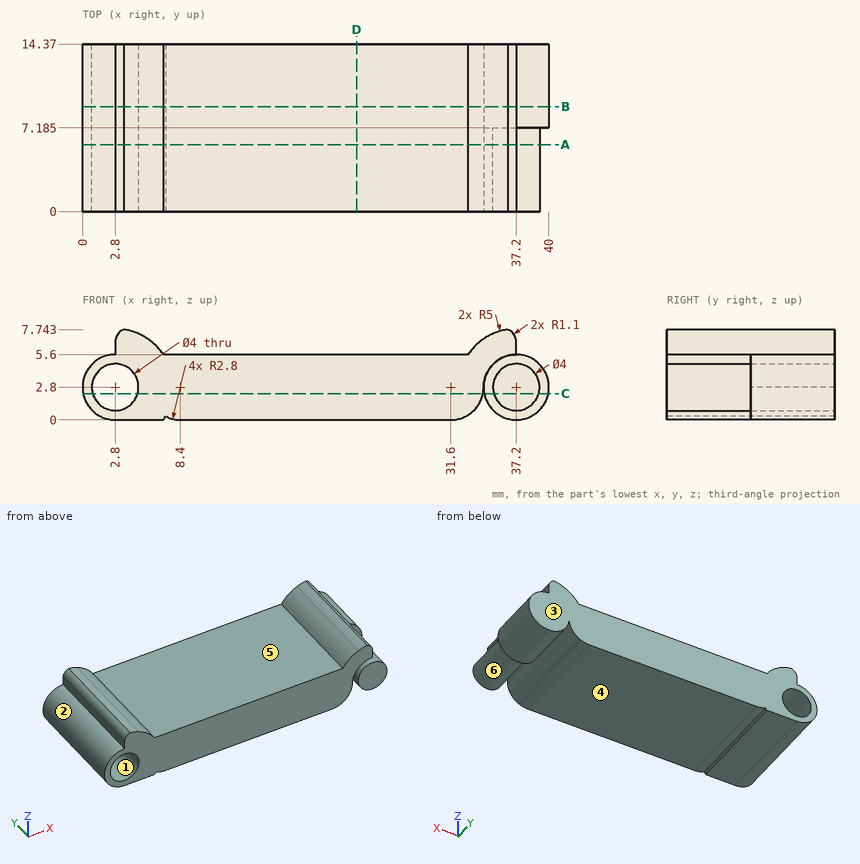
Could you check a few things on this drawing? It's one solid part, dimensions in mm from its lowest x, y, z. A direction names the side the tool comes from. Coordinates: 2 decimals unless noted, no trailing zeros. Write each loop counter-clockwise with the first axis right and the second up, starting at its lowest first coordinate (ties: lowest second). Pieces come first, ordered by that corner, then holes.
Q1. Which directions (+Z, -Z, +X, -X, +Y, -Y) give clear straight access to the entire face, cutting with the end or side of a thin tool? Please do the marked faces 4, 5 and 6.
Results found:
face 4: -Z, +X, -X, +Y, -Y
face 5: +Z, +Y, -Y
face 6: -Y
Q2. If we mould it in two halves opening along X, with no side actions, what happens to the marked faces 1, 2 and 3? For each: +X half, -X half, draft (parallel to the pull), parting line (faces both ways), or undercut.
Results found:
face 1: undercut
face 2: -X half
face 3: draft
Q3. Imagine slicing it at C-C, the plane z = 2.25. List the corners of the cut face in (x, y) for me (1 decimal), plus the area to 3 significant figures.
Results found:
outline: (0.1, 0) - (0.9, 0) - (0.9, 14.4) - (0.1, 14.4) - close; (4.7, 0) - (34.3, 0) - (34.3, 14.4) - (4.7, 14.4) - close; (34.5, 7.2) - (35.3, 7.2) - (35.3, 0) - (39.1, 0) - (39.1, 7.2) - (39.9, 7.2) - (39.9, 14.4) - (34.5, 14.4) - close
area: 505 mm2
Q4. Imagine slicing it at B-B, the plane y = 9. List the corners of the cut face in (x, z) for me.
Results found:
outline: (2.8, 0) - (6.94, 0) arc R5 ccw to (7.13, 0.3) arc R2.8 ccw to (8.4, 0) - (31.6, 0) arc R2.8 ccw to (34.4, 2.8) arc R2.8 ccw (long way) to (37.2, 5.6) - (37.2, 6.7) arc R1.1 ccw to (36.45, 7.74) arc R5 ccw to (33.06, 5.6) - (6.94, 5.6) arc R5 ccw to (3.55, 7.74) arc R1.1 ccw to (2.8, 6.7) - (2.8, 5.6) arc R2.8 ccw to start; hole circle Ø4 at (2.8, 2.8)
Q5. Imagine slicing it at D-D, the plane x = 23.5. List the corners of the cut face in (y, z) for me.
Results found:
outline: (0, 0) - (14.37, 0) - (14.37, 5.6) - (0, 5.6) - close
Q6. Imagine slicing it at A-A, the plane y = 5.75. List the corners of the cut face in (x, z) for me.
Results found:
outline: (2.8, 0) - (6.94, 0) arc R5 ccw to (7.13, 0.3) arc R2.8 ccw to (8.4, 0) - (31.6, 0) arc R2.8 ccw to (34.4, 2.8) arc R2.8 cw to (37.2, 5.6) - (37.2, 6.7) arc R1.1 ccw to (36.45, 7.74) arc R5 ccw to (33.06, 5.6) - (6.94, 5.6) arc R5 ccw to (3.55, 7.74) arc R1.1 ccw to (2.8, 6.7) - (2.8, 5.6) arc R2.8 ccw to start; circle Ø4 at (37.2, 2.8); hole circle Ø4 at (2.8, 2.8)
Q7. For P1, Ø2, axis at y = 12, z = 5, coming from the +X side; P2, Ø1.5, axis at x = 17, z = 6.5, coming from the -Y side; P3, Ø4, axis at y = 9.5, z = 5, coming from the -X side; P4, Ø0.9, axis at y = 4.5, z = 6, coming from the +X side, each with a flat end and sliding along its axis, tell me the tip position at first contact or that it passes through.
Results found:
P1: stops at x = 39.73
P2: passes through
P3: stops at x = 0.01
P4: stops at x = 37.2
Q8. Please list where these lines run through material, in increasing order: L1, parallel to X at y = 3, z = 2.75; L2, parallel to X at y = 9.5, z = 1.75 (1 decimal); L3, parallel to Z at x = 30.5, y = 2.5.
Results found:
L1: x = 0 to 0.8, 4.8 to 34.4, 35.2 to 39.2
L2: x = 0.2 to 1.1, 4.5 to 34.2, 34.6 to 39.8
L3: z = 0 to 5.6
